Can you work these out from the drawing? Everything is in mm from the part's minimum corner. Give positions to 0.01 mm unless a question says otherwise; leave off trailing zeros. Order: outer loops, then holes, each group sorted by start corner. A loop starts at its lowest first (then second) coordinate and runs counter-clockwise, first axis right, second up. Notation, with made-up numbers: (70, 44.5) - (86, 44.5) arc R22 ccw to (86, 62.5) - close; hole circle Ø9 at (85, -18.75). An arc over 180 degrees is marked (long way). One line per question, with ' | ' between items.
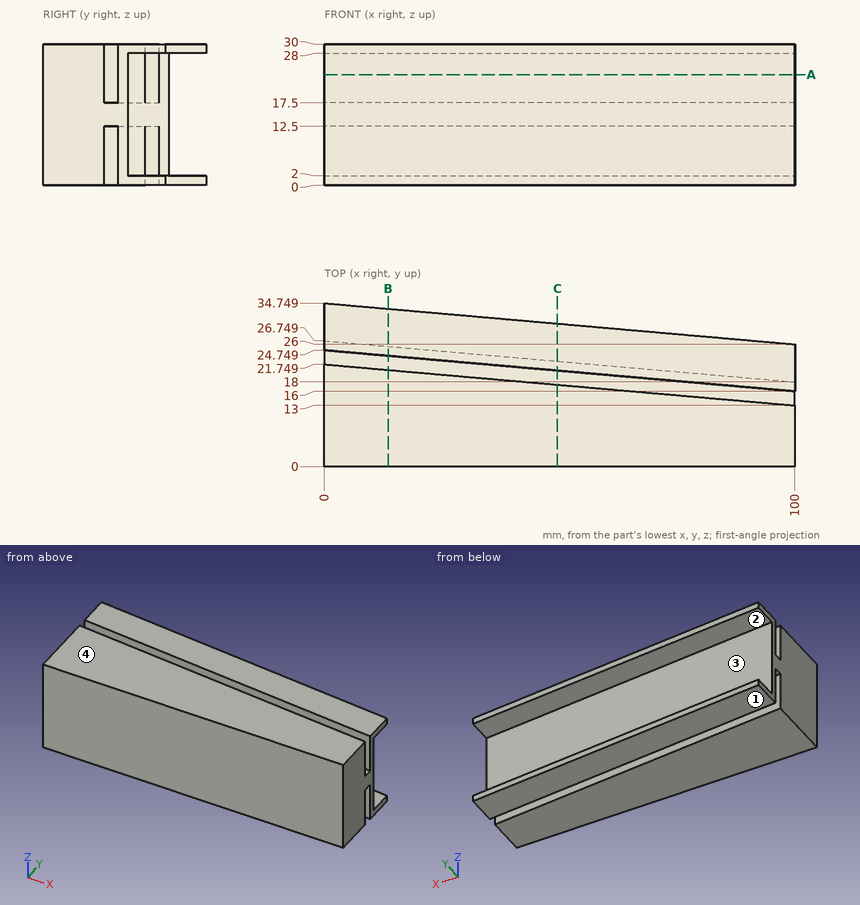
(1) If we mould it in two halves opening along Z, with no side actions, what happens to the marked faces 1, 2, 3 and 4? For each: released by +Z, released by -Z, zero draft, split by the parting line, or undercut.
Answer below:
face 1: released by -Z | face 2: undercut | face 3: undercut | face 4: released by +Z
(2) Imagine slicing it at B-B (x = 13.5). List the corners of the cut face in (y, z) for me.
Answer below:
outline: (0, 0) - (20.57, 0) - (20.57, 12.5) - (23.57, 12.5) - (23.57, 0) - (33.57, 0) - (33.57, 2) - (25.57, 2) - (25.57, 28) - (33.57, 28) - (33.57, 30) - (23.57, 30) - (23.57, 17.5) - (20.57, 17.5) - (20.57, 30) - (0, 30) - close
(3) Imagine slicing it at C-C (x = 49.5). List the corners of the cut face in (y, z) for me.
Answer below:
outline: (0, 0) - (17.42, 0) - (17.42, 12.5) - (20.42, 12.5) - (20.42, 0) - (30.42, 0) - (30.42, 2) - (22.42, 2) - (22.42, 28) - (30.42, 28) - (30.42, 30) - (20.42, 30) - (20.42, 17.5) - (17.42, 17.5) - (17.42, 30) - (0, 30) - close
(4) Will these pins go through, and if not, where does the flat tip stop? pin 1 (1.5 mm diameter, centred on x = 73, z = 15, fed in from -Y); pin 2 (8 mm diameter, centred on x = 36.5, z = 25, fed in from +Y); pin 3 (1.5 mm diameter, centred on x = 64.5, y = 31, fed in from +Z); pin 4 (6 mm diameter, centred on x = 46, z = 23.5, fed in from +Y).
Answer below:
pin 1: y = 0 | pin 2: y = 31.79 | pin 3: through | pin 4: y = 22.99
(5) Imagine slicing it at A-A (z = 23.5). List the corners of the cut face in (x, y) for me.
Answer below:
outline: (0, 0) - (100, 0) - (100, 13) - (0, 21.75) - close; (0, 24.75) - (100, 16) - (100, 18) - (0, 26.75) - close
(6) If I drill on line 1 (Z direction, x = 79, y = 20.5); line 2 (Z direction, x = 90, y = 16); line 3 (Y direction, x = 23.5, z = 8), over which ranges is the centre line in solid material (lowest first)?
Answer below:
line 1: 0 to 2, 28 to 30 | line 2: 12.5 to 17.5 | line 3: 0 to 19.69, 22.69 to 24.69
